```python
from build123d import *

# Parameters (mm, degrees)
SKETCH_1_R          = 1.95
SKETCH_1_R_2        = 7
EXTRUDE_1_DEPTH     = 4
SKETCH_2_R          = 2
CUT_EXTRUDE_1_DEPTH = 10
CUT_EXTRUDE_2_DEPTH = 10
FILLET_1_R          = 10


with BuildPart() as part:
    # 草图1 → 凸台-拉伸1 (new body)
    with BuildSketch(Plane.XY):
        with BuildLine():
            Line((-7.32233047, 7.32233047), (-107.32233047, 107.32233047))
            ThreePointArc((-107.32233047, 107.32233047), (-112.741649253, 134.567085809), (-89.644660941, 150))
            Line((-89.644660941, 150), (389.644660941, 150))
            ThreePointArc((389.644660941, 150), (412.741649253, 134.567085809), (407.32233047, 107.32233047))
            Line((407.32233047, 107.32233047), (307.32233047, 7.32233047))
            ThreePointArc((307.32233047, 7.32233047), (299.21174675, 1.903011687), (289.644660941, 0))
            Line((289.644660941, 0), (10.355339059, 0))
            ThreePointArc((10.355339059, 0), (0.78825325, 1.903011687), (-7.32233047, 7.32233047))
        make_face()
        with Locations((50.355339059, 125)):
            Circle(SKETCH_1_R, mode=Mode.SUBTRACT)
        with Locations((249.644660941, 125)):
            Circle(SKETCH_1_R, mode=Mode.SUBTRACT)
        with Locations((101.213203436, 15)):
            Circle(SKETCH_1_R, mode=Mode.SUBTRACT)
        with Locations((198.786796564, 15)):
            Circle(SKETCH_1_R, mode=Mode.SUBTRACT)
        with Locations((-89.644660941, 125)):
            Circle(SKETCH_1_R_2, mode=Mode.SUBTRACT)
        with Locations((6.213203436, 15)):
            Circle(SKETCH_1_R, mode=Mode.SUBTRACT)
        with Locations((293.786796564, 15)):
            Circle(SKETCH_1_R, mode=Mode.SUBTRACT)
        with Locations((389.644660941, 125)):
            Circle(SKETCH_1_R, mode=Mode.SUBTRACT)
    extrude(amount=EXTRUDE_1_DEPTH)

    # 草图2 → 切除-拉伸1 (cut)
    with BuildSketch(Plane.XY.offset(4)):
        with Locations((-10, 90)):
            Circle(SKETCH_2_R)
        with Locations((90, 90)):
            Circle(SKETCH_2_R)
        with Locations((210, 90)):
            Circle(SKETCH_2_R)
        with Locations((310, 90)):
            Circle(SKETCH_2_R)
        with Locations((-10, 70)):
            Circle(SKETCH_2_R)
        with Locations((90, 70)):
            Circle(SKETCH_2_R)
        with Locations((210, 70)):
            Circle(SKETCH_2_R)
        with Locations((310, 70)):
            Circle(SKETCH_2_R)
    extrude(amount=-CUT_EXTRUDE_1_DEPTH, mode=Mode.SUBTRACT)

    # 草图3 → 切除-拉伸2 (cut)
    with BuildSketch(Plane.XY.offset(4)):
        Polygon((28.213203436, 0), (40.213203436, 30), (67.213203436, 30), (79.213203436, 0), align=None)
        Polygon((123.213203436, 0), (135.213203436, 30), (164.786796564, 30), (176.786796564, 0), align=None)
        Polygon((220.786796564, 0), (232.786796564, 30), (259.786796564, 30), (271.786796564, 0), align=None)
    extrude(amount=-CUT_EXTRUDE_2_DEPTH, mode=Mode.SUBTRACT)

    # 圆角1
    fillet_1_edges = [part.edges().sort_by_distance(p)[0] for p in [
        (271.786796564, 0, 2),
        (220.786796564, 0, 2),
        (176.786796564, 0, 2),
        (123.213203436, 0, 2),
        (79.213203436, 0, 2),
        (28.213203436, 0, 2),
        (40.213203436, 30, 2),
        (67.213203436, 30, 2),
        (135.213203436, 30, 2),
        (164.786796564, 30, 2),
        (232.786796564, 30, 2),
        (259.786796564, 30, 2),
    ]]
    fillet(fillet_1_edges, radius=FILLET_1_R)


solid = part.part
```
Check sheet for the modelled part. Datum: model origin and axes. Units: mm. Round coordinates to 2 decimals unless told otherwise and drop trailing zeros. Loops run counter-clockwise (first coordinate to the right, second up) from the corner with the lowest first, then second, coordinate; pieces in that order, holes last. Notation, with made-up numbers: (32, 47) -> (75, 47) arc R28 ccw to (75, 76) -> close; hole circle Ø7 at (62, 81). An arc over 180 degrees is marked (long way). Write item = value, one per line. Start each with the question number.
1) Sectioned sample at A-A, the plane z = 1.5. State how many separate pieces and enclosed holes the cut face has, plus the area to 3 significant figures.
2) Gauge pin test, flat ends, axial feed: pin 1 Ø3.5 at (x, y) = (210, 90) entering from -Z; pin 2 Ø2 at (y, z) = (89, 3) entering from +X. Record the tip position at first contact, or that the pin passes through.
3) Thickness scan on probe 1 along Y at (x, z) = (210, 2.25); probe 2 along X at (y, z) = (17.5, 0.4); probe 3 along X at (y, z) = (29, 0.5). Record the ranges inside material, lowest first.
4) Sectioned sample at B-B, the plane y = 45. Record the cut outline in (x, z).
Results are:
q1.separate_pieces = 1
q1.enclosed_holes = 16
q1.area = 62,000 mm^2
q2.pin_1 = through
q2.pin_2 = 390
q3.probe_1 = 0 to 68, 72 to 88, 92 to 150
q3.probe_2 = -17.5 to 35.21, 72.21 to 130.21, 169.79 to 227.79, 264.79 to 317.5
q3.probe_3 = -29 to 42.62, 64.8 to 137.62, 162.38 to 235.2, 257.38 to 329
q4.outline = (-45, 0) -> (345, 0) -> (345, 4) -> (-45, 4) -> close
